from build123d import *

# Parameters (mm, degrees)
BASE_DEPTH           = 10
ESQUISSE5_R          = 2.5
VIDE_ACCES_VIS_DEPTH = 31.929020524


with BuildPart() as part:
    # Esquisse2 → BASE (new body)
    with BuildSketch(Plane(origin=(0, 0, 0), x_dir=(0, 0, -1), z_dir=(1, 0, 0))):
        with BuildLine():
            Line((-27.502803686, 10), (-14.361406616, 10))
            Line((-14.361406616, 10), (-12.502803686, 10))
            ThreePointArc((-12.502803686, 10), (0, 16.01), (12.502803686, 10))
            Line((12.502803686, 10), (14.361406616, 10))
            Line((14.361406616, 10), (22.502803686, 10))
            Line((22.502803686, 10), (27.502803686, 10))
            Line((27.502803686, 10), (27.502803686, 15))
            Line((27.502803686, 15), (13.24387028, 15))
            ThreePointArc((13.24387028, 15), (0, 20.01), (-13.24387028, 15))
            Line((-13.24387028, 15), (-27.502803686, 15))
            Line((-27.502803686, 15), (-27.502803686, 10))
        make_face()
    extrude(amount=BASE_DEPTH)

    # Esquisse5 → VIDE ACCES VIS (cut, through all)
    with BuildSketch(Plane.XZ.offset(-10)):
        with Locations(Location((5, 22.502803686, 0), (0, 0, 270))):
            Circle(ESQUISSE5_R)
        with Locations(Location((5, -22.502803686, 0), (0, 0, 270))):
            Circle(ESQUISSE5_R)
    extrude(amount=-VIDE_ACCES_VIS_DEPTH, mode=Mode.SUBTRACT)


solid = part.part
The listing builds one solid part. Answer for the finished solid, in the listing's coordinates (mm). A direction names the side the tool comes from. Coordinates: 2 decimals unless noted, no trailing zeros. Write each loop counter-clockwise with the first axis right and the second up, starting at its lowest first coordinate (ties: lowest second). Pieces come first, ordered by that corner, then holes. Notation, with made-up numbers: M 89.25,-3 L 142.25,-3 A24 ccw 142.25,9 Z; hole C 89,32 d5. An arc over 180 degrees is marked long. Put each result on its own line as item: value. Start each with the question number.
1. Flat-ended cylindrical pins translate along their axes: P1, Ø3, axis at x = 5, z = 19.5, coming from the +Y side; P2, Ø4, axis at x = 2, z = -11.5, coming from the -Y side; P3, Ø4, axis at x = 8, z = 2.5, coming from the +Y side; P4, Ø4, axis at x = 5, z = 13, coming from the +Y side. Find the tip coordinate at first contact, or state that the pin passes through.
2. A cutting plane is placed at A-A on y = 13. Write down the section's boundary in (x, z).
3. For a pull along Z with two mould halves and no side action, classify faces 1 (the flat face through (6, 10, 20)), 2 (the cylindrical face through (4.93, 20.01, -0.2)), 3 (the cylindrical face through (4.93, 16.01, 0.2)) as pulls with the +Z half, pulls with the -Z half, needs draft (parallel to the pull), parting line crosses it, or undercut.
4. Which of the six approach directions +Z, -Z, +X, -X, +Y, -Y give full straight-line access (tool end or side, diameter ignored) to faces 4 (the flat face through (4, 15, 20)), 5 (the flat face through (5, 15, -19)), 6 (the flat face through (10, 16.2, 0.4))?
5. A cutting plane is placed at D-D on x = 1. Write down the section's boundary in (y, z).
6. A cutting plane is placed at C-C on x = 5. Write down the section's boundary in (y, z).
7. A cutting plane is placed at B-B on z = -22. Write down the section's boundary in (x, y), then the cut area to 3 significant figures.
8. Consider line 1 (Y direction, x = 8.25, z = 22); line 2 (Z direction, x = 1, y = 11.25); line 3 (Z direction, x = 3.5, y = 13). Determine where each line is inside the solid, lowest interval first. Write a range as from..to.
Resolved:
1. P1: stops at y = 15
1. P2: stops at y = 10
1. P3: stops at y = 20
1. P4: stops at y = 16.72
2. outline: M 0,-27.5 L 10,-27.5 L 10,-9.34 L 0,-9.34 Z; M 0,9.34 L 10,9.34 L 10,27.5 L 0,27.5 Z; hole C 5,-22.5 d5; hole C 5,22.5 d5
3. face 1: needs draft
3. face 2: parting line crosses it
3. face 3: undercut
4. face 4: +Z, +X, -X, +Y
4. face 5: -Z, +X, -X, +Y
4. face 6: +Z, -Z, +X, +Y, -Y
5. outline: M 10,-27.5 L 15,-27.5 L 15,-13.24 A20.01 ccw 15,13.24 L 15,27.5 L 10,27.5 L 10,12.5 A16.01 cw 10,-12.5 Z
6. outline: M 10,-27.5 L 15,-27.5 L 15,-25 L 10,-25 Z; M 10,-20 L 15,-20 L 15,-13.24 A20.01 ccw 15,13.24 L 15,20 L 10,20 L 10,12.5 A16.01 cw 10,-12.5 Z; M 10,25 L 15,25 L 15,27.5 L 10,27.5 Z
7. outline: M 0,10 L 2.55,10 L 2.55,15 L 0,15 Z; M 7.45,10 L 10,10 L 10,15 L 7.45,15 Z
7. area: 25.5 mm2
8. line 1: y = 10..15
8. line 2: z = -27.5..-11.39, 11.39..27.5
8. line 3: z = -27.5..-24.5, -20.5..-9.34, 9.34..20.5, 24.5..27.5
